```python
from build123d import *

# Parameters (mm, degrees)
BOSS_EXTRUDE1_DEPTH = 6


with BuildPart() as part:
    # Sketch1 → Boss-Extrude1 (new body)
    with BuildSketch(Plane.XY):
        Polygon((-506.545769475, -193.251863484), (-506.545769475, -169.651863484), (-451.545769475, -169.651863484), (-451.545769475, -193.251863484), (-467.945769475, -193.251863484), (-467.945769475, -189.751863484), (-468.150214517, -188.198949213), (-468.749617052, -186.751863484), (-469.703128788, -185.509222797), (-470.945769475, -184.555711061), (-472.392855205, -183.956308526), (-473.945769475, -183.751863484), (-475.498683746, -183.956308526), (-476.945769475, -184.555711061), (-478.188410162, -185.509222797), (-479.141921898, -186.751863484), (-479.741324433, -188.198949213), (-479.945769475, -189.751863484), (-479.945769475, -193.251863484), align=None)
        Polygon((-455.545769475, -190.551863484), (-455.079895194, -190.490529971), (-454.645769475, -190.310709211), (-454.272977269, -190.02465569), (-453.986923748, -189.651863484), (-453.807102988, -189.217737765), (-453.745769475, -188.751863484), (-453.807102988, -188.285989203), (-453.986923748, -187.851863484), (-454.272977269, -187.479071278), (-454.645769475, -187.193017757), (-455.079895194, -187.013196996), (-455.545769475, -186.951863484), (-456.011643756, -187.013196996), (-456.445769475, -187.193017757), (-456.818561681, -187.479071278), (-457.104615202, -187.851863484), (-457.284435962, -188.285989203), (-457.345769475, -188.751863484), (-457.284435962, -189.217737765), (-457.104615202, -189.651863484), (-456.818561681, -190.02465569), (-456.445769475, -190.310709211), (-456.011643756, -190.490529971), align=None, mode=Mode.SUBTRACT)
        Polygon((-502.079895194, -190.490529971), (-501.645769475, -190.310709211), (-501.272977269, -190.02465569), (-500.986923748, -189.651863484), (-500.807102988, -189.217737765), (-500.745769475, -188.751863484), (-500.807102988, -188.285989203), (-500.986923748, -187.851863484), (-501.272977269, -187.479071278), (-501.645769475, -187.193017757), (-502.079895194, -187.013196996), (-502.545769475, -186.951863484), (-503.011643756, -187.013196996), (-503.445769475, -187.193017757), (-503.818561681, -187.479071278), (-504.104615202, -187.851863484), (-504.284435962, -188.285989203), (-504.345769475, -188.751863484), (-504.284435962, -189.217737765), (-504.104615202, -189.651863484), (-503.818561681, -190.02465569), (-503.445769475, -190.310709211), (-503.011643756, -190.490529971), (-502.545769475, -190.551863484), align=None, mode=Mode.SUBTRACT)
        Polygon((-492.445769475, -186.153787272), (-492.482936855, -186.153787272), (-493.067089819, -186.63054314), (-493.104257199, -186.63054314), (-493.581013066, -187.251863484), (-493.880714334, -187.975406348), (-493.982936855, -188.751863484), (-493.880714334, -189.528320619), (-493.581013066, -190.251863484), (-493.104257199, -190.873183827), (-492.482936855, -191.349939695), (-491.75939399, -191.649640963), (-490.982936855, -191.751863484), (-490.20647972, -191.649640963), (-489.482936855, -191.349939695), (-488.861616511, -190.873183827), (-488.384860644, -190.251863484), (-488.085159376, -189.528320619), (-487.982936855, -188.751863484), (-488.085159376, -187.975406348), (-488.384860644, -187.251863484), (-488.861616511, -186.63054314), (-489.445769475, -186.153787272), (-489.482936855, -186.153787272), (-490.16931234, -185.854086005), (-490.20647972, -185.854086005), (-490.945769475, -185.751863484), (-490.982936855, -185.751863484), (-491.72222661, -185.854086005), (-491.75939399, -185.854086005), align=None, mode=Mode.SUBTRACT)
    extrude(amount=BOSS_EXTRUDE1_DEPTH)


solid = part.part
```
Can you work these out from the model? Positions are in its coordinate system, mm. A direction names the side the tool comes from. Give positions to 0.01 mm unless a question says otherwise; leave off trailing zeros. Write item = value, one per line. Start each with the question number.
Q1. I need wall thicknesses on probe 1 along X at (y, z) = (-186.5, 3.3); probe 2 along X at (y, z) = (-191, 3.4); probe 3 along Y at (x, z) = (-454.5, 1.2). Which ranges of each line are inside material? Lowest first, please. Write a range as [from, to].
Q2. Suppose I cut it at A-A (z = 4). Count the separate pieces of the cut face and the enclosed holes in it, plus the area to 3 significant figures.
Q3. We'd pull the mould along X, two halves only. Please class faces 1 (the flat face through (-467.946, -192, 3)), 2 (the flat face through (-479, -181, 0)), 3 (the flat face through (-506.546, -182, 3)): pulls with the +X half, pulls with the -X half, needs draft (parallel to the pull), parting line crosses it, or undercut.
Q4. For faces 4 (the flat face through (-479.946, -191, 3)), 5 (the flat face through (-493, -193.252, 3)), which set-ups out of +Z, -Z, +X, -X, +Y, -Y let a thin tool reach every point of the face, with its end or its side?
Check result:
q1.probe_1 = [-506.55, -492.91], [-489.02, -478.95], [-468.94, -451.55]
q1.probe_2 = [-506.55, -492.94], [-489.03, -479.95], [-467.95, -451.55]
q1.probe_3 = [-193.25, -190.2], [-187.3, -169.65]
q2.separate_pieces = 1
q2.enclosed_holes = 3
q2.area = 1,150 mm2
q3.face_1 = undercut
q3.face_2 = needs draft
q3.face_3 = pulls with the -X half
q4.face_4 = +Z, -Z, -Y
q4.face_5 = +Z, -Z, +X, -X, -Y
